Check sheet for the modelled part. Datum: model origin and axes. Units: mm. Give positions to 0.01 mm unless a question says otherwise; leave off trailing zeros. Order: outer loops, then holes, each group sorted by start corner. A loop starts at its lowest first (then second) coordinate and runs counter-clockwise, first axis right, second up. Notation, with made-up numbers: (30.25, 2.25) -> (84.25, 2.25) arc R19 cw to (84.25, 13.25) -> close; hole circle Ø2 at (40.25, -22). An arc over 180 degrees is marked (long way). Write each question's results on one line, items separated by ' | '.
from build123d import *

# Parameters (mm, degrees)
BOX001_W               = 7
BOX001_H               = 20
BOX001_DEPTH           = 7
BOX001_PLACEMENT_ANGLE = 45
BOX_W                  = 10
BOX_H                  = 20
BOX_DEPTH              = 10


with BuildPart() as cube001:
    # Box001 → Box001 (new body)
    with BuildSketch(Plane.XY):
        with Locations((3.5, 10)):
            Rectangle(BOX001_W, BOX001_H)
    extrude(amount=BOX001_DEPTH)


with BuildPart() as cube001_1:
    # Box001 placement: moved
    add(cube001.part.moved(Location((-0.0011, 0, 10))).rotate(Axis((-0.0011, 0, 10), (0, 1, 0)), BOX001_PLACEMENT_ANGLE))


with BuildPart() as fusion:
    # Box → Box (new body)
    with BuildSketch(Plane.XY):
        with Locations((5, 10)):
            Rectangle(BOX_W, BOX_H)
    extrude(amount=BOX_DEPTH)

    # Fusion: union Cube001
    add(cube001_1.part)


with BuildPart() as fusion_1:
    # Fusion placement: moved
    add(fusion.part.moved(Location((-5, -10, 0))))


solid = fusion_1.part
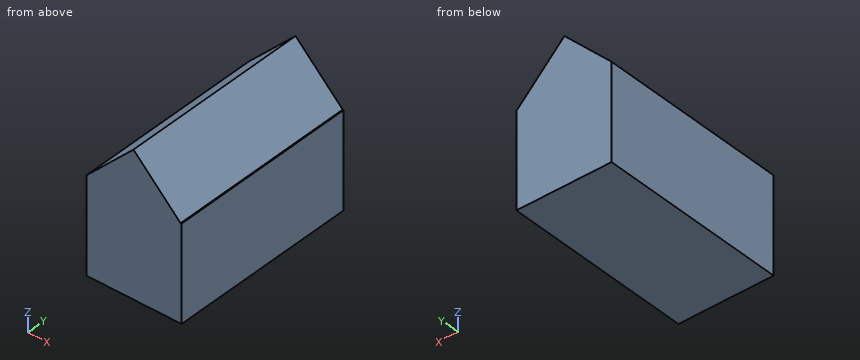
1. Section check C-C on z = 11. Record the cut outline in (x, y), then the cut area to 3 significant figures.
Verdict:
outline: (-4, -10) -> (3.9, -10) -> (3.9, 10) -> (-4, 10) -> close | area: 158 mm^2
2. Material ranges on probe 1 along X at (y, z) = (-4.5, 2.5); probe 2 along Z at (x, y) = (4.25, 6.5); probe 3 along X at (y, z) = (2.5, 11.25), recorded low to high. Write a range as from..to.
Verdict:
probe 1: x = -5..5 | probe 2: z = 0..10.65 | probe 3: x = -3.75..3.65
3. Section check B-B on x = -2.25. Record the cut outline in (y, z), then the cut area to 3 significant figures.
Verdict:
outline: (-10, 0) -> (10, 0) -> (10, 12.75) -> (-10, 12.75) -> close | area: 255 mm^2
4. Gauge pin test, flat ends, axial feed: pin 1 Ø2 at (y, z) = (-2.5, 12.5) entering from -X; pin 2 Ø3 at (x, y) = (1, 2.5) entering from +Z. Record the tip position at first contact, or that the pin passes through.
Verdict:
pin 1: stops at x = -3.5 | pin 2: stops at z = 14.95
